```python
from build123d import *

# Parameters (mm, degrees)
F1_DEPTH = 1
F2_DEPTH = 10


with BuildPart() as f1:
    # F0 (on Top) → F1 (new body)
    with BuildSketch(Plane.XY):
        with BuildLine():
            Line((0, 10), (0, 50))
            Line((0, 50), (-5, 50))
            Line((-5, 50), (-5, 20))
            Line((-5, 20), (-15, 20))
            Line((-15, 20), (-25, 20))
            Line((-25, 20), (-25, 50))
            Line((-25, 50), (-55, 30))
            Line((-55, 30), (-35, 30))
            Line((-35, 30), (-35, 10))
            Line((-35, 10), (-35, 0.120711))
            ThreePointArc((-35, 0.120711), (-34.964645, 0.035355), (-34.879289, 0))
            Line((-34.879289, 0), (-25, 0))
            Line((-25, 0), (-25, 10))
            Line((-25, 10), (0, 10))
        make_face()
        Polygon((-5, 20), (-5, 50), (-25, 50), (-25, 20), (-15, 20), align=None)
        with BuildLine():
            Line((-35.120711, 0), (-55, 0))
            Line((-55, 0), (-45, -40))
            Line((-45, -40), (-45, -10))
            Line((-45, -10), (-35, -10))
            Line((-35, -10), (-35, -0.120711))
            ThreePointArc((-35, -0.120711), (-35.035355, -0.035355), (-35.120711, 0))
        make_face()
        with BuildLine():
            Line((0, -50), (0, 10))
            Line((0, 10), (-25, 10))
            Line((-25, 10), (-25, 0))
            Line((-25, 0), (-34.879289, 0))
            ThreePointArc((-34.879289, 0), (-34.964645, 0.035355), (-35, 0.120711))
            Line((-35, 0.120711), (-35, 10))
            Line((-35, 10), (-35, 30))
            Line((-35, 30), (-55, 30))
            Line((-55, 30), (-55, 0))
            Line((-55, 0), (-35.120711, 0))
            ThreePointArc((-35.120711, 0), (-35.035355, -0.035355), (-35, -0.120711))
            Line((-35, -0.120711), (-35, -10))
            Line((-35, -10), (-45, -10))
            Line((-45, -10), (-45, -40))
            Line((-45, -40), (-35, -40))
            Line((-35, -40), (-35, -50))
            Line((-35, -50), (0, -50))
        make_face()
    extrude(amount=-F1_DEPTH)

    # F0 (on Top) → F2 (join)
    with BuildSketch(Plane.XY):
        Polygon((-5, 20), (-5, 50), (-25, 50), (-25, 20), (-15, 20), align=None)
        with BuildLine():
            Line((0, -50), (0, 10))
            Line((0, 10), (-25, 10))
            Line((-25, 10), (-25, 0))
            Line((-25, 0), (-34.879289, 0))
            ThreePointArc((-34.879289, 0), (-34.964645, 0.035355), (-35, 0.120711))
            Line((-35, 0.120711), (-35, 10))
            Line((-35, 10), (-35, 30))
            Line((-35, 30), (-55, 30))
            Line((-55, 30), (-55, 0))
            Line((-55, 0), (-35.120711, 0))
            ThreePointArc((-35.120711, 0), (-35.035355, -0.035355), (-35, -0.120711))
            Line((-35, -0.120711), (-35, -10))
            Line((-35, -10), (-45, -10))
            Line((-45, -10), (-45, -40))
            Line((-45, -40), (-35, -40))
            Line((-35, -40), (-35, -50))
            Line((-35, -50), (0, -50))
        make_face()
    extrude(amount=F2_DEPTH)

    # F3: F1 across plane


with BuildPart() as f1_1:
    add(f1.part)
    add(f1.part.mirror(Plane.YZ))


solid = f1_1.part
```
The listing builds one solid part. Answer for the finished solid, in the listing's coordinates (mm). A direction names the side the tool comes from. Round coordinates to 2 decimals unless told otherwise and drop trailing zeros. Loops run counter-clockwise (first coordinate to the right, second up) from the corner with the lowest first, then second, coordinate; pieces in that order, holes last.
1) A cutting plane is placed at A-A on y = 6. Determine the outline of the cut face in (x, z), plus the area to 3 significant figures.
Outcome:
outline: (-55, -1) - (55, -1) - (55, 10) - (35, 10) - (35, 0) - (25, 0) - (25, 10) - (-25, 10) - (-25, 0) - (-35, 0) - (-35, 10) - (-55, 10) - close
area: 1,010 mm2
2) A cutting plane is placed at D-D on x = -0.5. Determine the outline of the cut face in (y, z), plus the area to 3 significant figures.
Outcome:
outline: (-50, -1) - (50, -1) - (50, 0) - (10, 0) - (10, 10) - (-50, 10) - close
area: 700 mm2
3) Consider line 1 (X direction, y = 20.5, z = 8.25); line 2 (X direction, y = 8, z = 9); line 3 (Y direction, x = -7.5, z = 7). Determine where each line is inside the solid, lowest interval first.
Outcome:
line 1: x = -55 to -35, -25 to -5, 5 to 25, 35 to 55
line 2: x = -55 to -35, -25 to 25, 35 to 55
line 3: y = -50 to 10, 20 to 50
4) For a pull along Y with two mould halves and no side action, classify faces 1 (the face through (55, 15, 4)), 2 (the face through (-40, -40, 5)), 3 (the face through (0, 10, 5)) as released by +Y, released by -Y, zero draft, split by the parting line, or undercut.
Outcome:
face 1: zero draft
face 2: released by -Y
face 3: undercut
5) Given P1, Ø3, axis at x = -44, z = 3.5, coming from the -Y side; P2, Ø3, axis at y = -7, z = 6.5, coming from the -X side; P3, Ø3, axis at x = 30, z = 3, coming from the +Y side, each flat-ended and moving along its own axis, determine where each tip first touches the part or whether it passes through.
Outcome:
P1: stops at y = -40
P2: stops at x = -35
P3: stops at y = 0
6) A cutting plane is placed at B-B on x = 14. Determine the outline of the cut face in (y, z), plus the area to 3 significant figures.
Outcome:
outline: (-50, -1) - (50, -1) - (50, 10) - (20, 10) - (20, 0) - (10, 0) - (10, 10) - (-50, 10) - close
area: 1,000 mm2
7) A cutting plane is placed at C-C on z = 6.25. Give the number of separate pieces and of enclosed holes in the cut face, plus the area to 3 significant figures.
Outcome:
separate pieces: 3
enclosed holes: 0
area: 7,000 mm2
8) For faces 4 (the face through (25, 5, 5)), 5 (the face through (-40, -10, 5)), 6 (the face through (40, -10, 5)), determine the directions among +Z, -Z, +X, -X, +Y, -Y from which every point of the face is accessible in a straight line to the end or side of a thin tool.
Outcome:
face 4: +Z, +Y
face 5: +Z, -X
face 6: +Z, +X
